Geometry check sheet. Reference: the model listing, model coordinates, mm. Face numbers are marked on the shaded views. A direction names the side the tool comes from. Coordinates: 2 decimals unless noted, no trailing zeros. Loops run counter-clockwise (first coordinate to the right, second up) from the corner with the lowest first, then second, coordinate; pieces in that order, holes last.
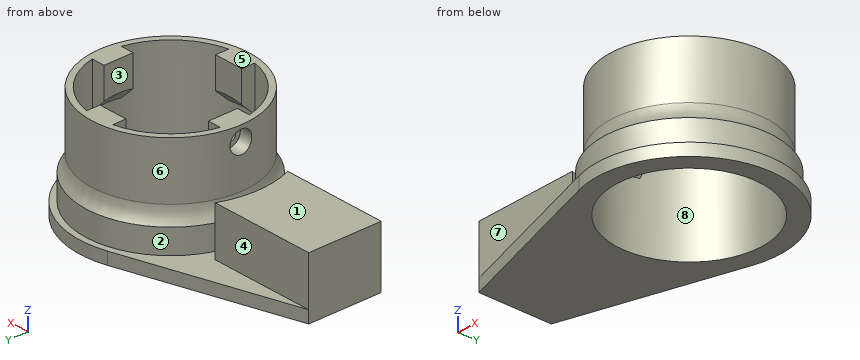
from build123d import *

# Parameters (mm, degrees)
ESQUISSE1_R                  = 30
BOSS_EXTRU_1_DEPTH           = 5
ESQUISSE6_R                  = 35
ESQUISSE6_R_2                = 30
BOSS_EXTRU_6_DEPTH           = 10
ESQUISSE7_R                  = 32.5
ESQUISSE7_R_2                = 30
BOSS_EXTRU_8_DEPTH           = 30
CONG_2_R                     = 10
BOSS_EXTRU_9_DEPTH           = 20
ESQUISSE9_W                  = 8
ESQUISSE9_H                  = 12
ESQUISSE9_W_2                = 12
ESQUISSE9_H_2                = 8
BOSS_EXTRU_10_DEPTH          = 12
CHANFREIN1_SIZE              = 6
ENL_V_MAT_EXTRU_1_REACH      = 86.89
ENL_V_MAT_EXTRU_1_END_RADIUS = 32.5
ESQUISSE10_R                 = 4.5
ESQUISSE12_R                 = 4.5
ESQUISSE12_R_2               = 2.6
BOSS_EXTRU_11_DEPTH          = 3


with BuildPart() as part:
    # Esquisse1 → Boss.-Extru.1 (new body)
    with BuildSketch(Plane.XY):
        with BuildLine():
            Line((-10.847469364, 35.896830061), (-80, 15))
            Line((-80, 15), (-80, -15))
            Line((-80, -15), (-10.847469364, -35.896830061))
            ThreePointArc((-10.847469364, -35.896830061), (37.5, 0), (-10.847469364, 35.896830061))
        make_face()
        Circle(ESQUISSE1_R, mode=Mode.SUBTRACT)
    extrude(amount=BOSS_EXTRU_1_DEPTH)

    # Esquisse6 → Boss.-Extru.6 (add)
    with BuildSketch(Plane.XY.offset(5)):
        Circle(ESQUISSE6_R)
        Circle(ESQUISSE6_R_2, mode=Mode.SUBTRACT)
    extrude(amount=BOSS_EXTRU_6_DEPTH)

    # Esquisse7 → Boss.-Extru.8 (add)
    with BuildSketch(Plane.XY.offset(15)):
        Circle(ESQUISSE7_R)
        Circle(ESQUISSE7_R_2, mode=Mode.SUBTRACT)
    extrude(amount=BOSS_EXTRU_8_DEPTH)

    # Congé2
    # the kernel refuses this fillet: 10 mm, written as the material it adds along each edge
    with BuildSketch(Plane(origin=(0, 0, 15), x_dir=(1, 0, 0), z_dir=(0, -1, 0))) as cong_2_piece_1:
        with BuildLine():
            CenterArc((42.5, 6.614378278), CONG_2_R, 180, 41.409622109)
            Line((32.5, 6.614378278), (32.3, 6.614378278))
            Line((32.3, 6.614378278), (32.3, 0))
            Line((32.3, 0), (32.5, -0.2))
            ThreePointArc((32.5, -0.2), (33.75, -0.2), (34.85, -0.132287566))
            Line((34.85, -0.132287566), (35, 0))
        make_face()
    revolve(axis=Axis((0, 0, 15), (0, 0, 1)))

    # Esquisse8 → Boss.-Extru.9 (add)
    with BuildSketch(Plane.XY.offset(5)):
        with BuildLine():
            Line((-80, 15), (-37.080992435, 15))
            ThreePointArc((-37.080992435, 15), (-40, 0), (-37.080992435, -15))
            Line((-37.080992435, -15), (-80, -15))
            Line((-80, -15), (-80, 15))
        make_face()
    extrude(amount=BOSS_EXTRU_9_DEPTH)

    # Esquisse9 → Boss.-Extru.10 (add)
    with BuildSketch(Plane.XY.offset(45)):
        with Locations((-27.941352507, 0)):
            Rectangle(ESQUISSE9_W, ESQUISSE9_H)
        with Locations((0, 27.941352507)):
            Rectangle(ESQUISSE9_W_2, ESQUISSE9_H_2)
        with Locations((27.941352507, 0)):
            Rectangle(ESQUISSE9_W, ESQUISSE9_H)
        with Locations((0, -27.941352507)):
            Rectangle(ESQUISSE9_W_2, ESQUISSE9_H_2)
    extrude(amount=-BOSS_EXTRU_10_DEPTH)

    # Chanfrein1
    # the kernel refuses this chamfer: 6 mm, written as the material it adds along each edge
    with BuildSketch(Plane(origin=(0, 0, 33), x_dir=(-0.6561519302770997, 0.75462881232672, 0), z_dir=(-0.75462881232672, -0.6561519302770997, 0))) as chanfrein1_piece_1_section:
        Polygon((30, CHANFREIN1_SIZE), (30 - CHANFREIN1_SIZE, 0), (30, 0), align=None)
    chanfrein1_piece_1 = revolve(axis=Axis((0, 0, 33), (0, 0, -1)), revolution_arc=82.01410645, mode=Mode.PRIVATE)
    chanfrein1_piece_1 = split(chanfrein1_piece_1, bisect_by=Plane(origin=(-6, 27.82841678, 31.008979001), z_dir=(1, 0, 0)), keep=Keep.TOP, mode=Mode.PRIVATE)
    chanfrein1_piece_1 = split(chanfrein1_piece_1, bisect_by=Plane(origin=(6, 27.82841678, 31.008979001), z_dir=(-1, 0, 0)), keep=Keep.TOP, mode=Mode.PRIVATE)
    chanfrein1_piece_1 = split(chanfrein1_piece_1, bisect_by=Plane(origin=(0, 23.941352507, 31.008979001), z_dir=(0, 1, 0)), keep=Keep.TOP, mode=Mode.PRIVATE)
    add(chanfrein1_piece_1)
    with BuildSketch(Plane(origin=(0, 0, 33), x_dir=(0.754635493716526, 0.6561442460490032, 0), z_dir=(-0.6561442460490032, 0.754635493716526, 0))) as chanfrein1_piece_2_section:
        Polygon((30, CHANFREIN1_SIZE), (30 - CHANFREIN1_SIZE, 0), (30, 0), align=None)
    chanfrein1_piece_2 = revolve(axis=Axis((0, 0, 33), (0, 0, -1)), revolution_arc=41.006469797, mode=Mode.PRIVATE)
    chanfrein1_piece_2 = split(chanfrein1_piece_2, bisect_by=Plane(origin=(27.828416771, 6, 31.008979004), z_dir=(0, -1, 0)), keep=Keep.TOP, mode=Mode.PRIVATE)
    chanfrein1_piece_2 = split(chanfrein1_piece_2, bisect_by=Plane(origin=(23.941352507, 3.002348554, 31.008979004), z_dir=(1, 0, 0)), keep=Keep.TOP, mode=Mode.PRIVATE)
    add(chanfrein1_piece_2)
    with BuildSketch(Plane(origin=(0, 0, 33), x_dir=(0.6561519302770998, -0.7546288123267199, 0), z_dir=(0.7546288123267199, 0.6561519302770998, 0))) as chanfrein1_piece_3_section:
        Polygon((30, CHANFREIN1_SIZE), (30 - CHANFREIN1_SIZE, 0), (30, 0), align=None)
    chanfrein1_piece_3 = revolve(axis=Axis((0, 0, 33), (0, 0, -1)), revolution_arc=82.01410645, mode=Mode.PRIVATE)
    chanfrein1_piece_3 = split(chanfrein1_piece_3, bisect_by=Plane(origin=(6, -27.82841678, 31.008979001), z_dir=(-1, 0, 0)), keep=Keep.TOP, mode=Mode.PRIVATE)
    chanfrein1_piece_3 = split(chanfrein1_piece_3, bisect_by=Plane(origin=(-6, -27.82841678, 31.008979001), z_dir=(1, 0, 0)), keep=Keep.TOP, mode=Mode.PRIVATE)
    chanfrein1_piece_3 = split(chanfrein1_piece_3, bisect_by=Plane(origin=(0, -23.941352507, 31.008979001), z_dir=(0, -1, 0)), keep=Keep.TOP, mode=Mode.PRIVATE)
    add(chanfrein1_piece_3)
    with BuildSketch(Plane(origin=(0, 0, 33), x_dir=(-0.7546288123267202, -0.6561519302770997, 0), z_dir=(0.6561519302770997, -0.7546288123267202, 0))) as chanfrein1_piece_4_section:
        Polygon((30, CHANFREIN1_SIZE), (30 - CHANFREIN1_SIZE, 0), (30, 0), align=None)
    chanfrein1_piece_4 = revolve(axis=Axis((0, 0, 33), (0, 0, -1)), revolution_arc=82.01410645, mode=Mode.PRIVATE)
    chanfrein1_piece_4 = split(chanfrein1_piece_4, bisect_by=Plane(origin=(-27.82841678, -6, 31.008979), z_dir=(0, 1, 0)), keep=Keep.TOP, mode=Mode.PRIVATE)
    chanfrein1_piece_4 = split(chanfrein1_piece_4, bisect_by=Plane(origin=(-27.82841678, 6, 31.008979), z_dir=(0, -1, 0)), keep=Keep.TOP, mode=Mode.PRIVATE)
    chanfrein1_piece_4 = split(chanfrein1_piece_4, bisect_by=Plane(origin=(-23.941352507, 0, 31.008979), z_dir=(-1, 0, 0)), keep=Keep.TOP, mode=Mode.PRIVATE)
    add(chanfrein1_piece_4)
    with BuildSketch(Plane(origin=(0, 0, 33), x_dir=(1, 0, 0), z_dir=(0, 1, 0))) as chanfrein1_piece_5_section:
        Polygon((30, CHANFREIN1_SIZE), (30 - CHANFREIN1_SIZE, 0), (30, 0), align=None)
    chanfrein1_piece_5 = revolve(axis=Axis((0, 0, 33), (0, 0, -1)), revolution_arc=41.006469797, mode=Mode.PRIVATE)
    chanfrein1_piece_5 = split(chanfrein1_piece_5, bisect_by=Plane(origin=(27.828416774, -6, 31.008979003), z_dir=(0, 1, 0)), keep=Keep.TOP, mode=Mode.PRIVATE)
    chanfrein1_piece_5 = split(chanfrein1_piece_5, bisect_by=Plane(origin=(23.941352507, -3.002348554, 31.008979003), z_dir=(1, 0, 0)), keep=Keep.TOP, mode=Mode.PRIVATE)
    add(chanfrein1_piece_5)

    # Enlèv. mat.-Extru.1: up to this cylinder (the profile starts inside it)
    enl_v_mat_extru_1_end = Plane(origin=(0, 0, 39), z_dir=(0, 0, -1)) * Cylinder(ENL_V_MAT_EXTRU_1_END_RADIUS, 239.78, mode=Mode.PRIVATE)
    # Esquisse10 → Enlèv. mat.-Extru.1 (cut, up to the surface)
    with BuildSketch(Plane(origin=(-23.941352507, 0, 0), x_dir=(0, 0, -1), z_dir=(1, 0, 0)), mode=Mode.PRIVATE) as enl_v_mat_extru_1_sk1:
        with Locations((-39, 0)):
            Circle(ESQUISSE10_R)
    enl_v_mat_extru_1_tool1 = extrude(enl_v_mat_extru_1_sk1.sketch, amount=-ENL_V_MAT_EXTRU_1_REACH, mode=Mode.PRIVATE) & enl_v_mat_extru_1_end
    add(enl_v_mat_extru_1_tool1.solids().sort_by_distance((-23.941353, 0, 39))[0], mode=Mode.SUBTRACT)

    # Esquisse12 → Boss.-Extru.11 (add)
    with BuildSketch(Plane(origin=(-23.941352507, 0, 0), x_dir=(0, 0, -1), z_dir=(1, 0, 0))):
        with Locations((-39, 0)):
            Circle(ESQUISSE12_R)
        with Locations((-39, 0)):
            Circle(ESQUISSE12_R_2, mode=Mode.SUBTRACT)
    extrude(amount=-BOSS_EXTRU_11_DEPTH)


solid = part.part
(1) Sectioned sample at B-B on z = 7. Record the cut outline in (x, y), and give its area (3 significant figures).
Findings:
outline: (-80, -15) - (-37.08, -15) arc R40 cw to (-37.08, 15) - (-80, 15) - close; circle Ø70 at (0, 0); hole circle Ø60 at (0, 0)
area: 2,250 mm2
(2) Access from +Z, -Z, +X, -X, +Y, -Y to the whole of each face (thin tool, end or side, straight path). Record for the marked faces 1, 2, 3 and 4.
Findings:
face 1: +Z, -X, +Y, -Y
face 2: +Z
face 3: +Z, -Z
face 4: +Z, -X, +Y
(3) Scan lines: L1, parallel to X at y = -10.5, z = 9; L2, parallel to Y at x = 0, z = 14; L3, parallel to X at y = -2, z = 23. Record each from-to range of solid material in increasing order.
Findings:
L1: x = -80 to -38.6, -33.39 to -28.1, 28.1 to 33.39
L2: y = -35 to -30, 30 to 35
L3: x = -80 to -39.95, -32.44 to -29.93, 29.93 to 32.44
(4) Sectioned sample at C-C on z = 39. Record the cut outline in (x, y), and give its area (3 significant figures).
Findings:
outline: (-32.19, -4.5) arc R32.5 ccw (long way) to (-32.19, 4.5) - (-26.94, 4.5) - (-26.94, 2.6) - (-23.94, 2.6) - (-23.94, 6) - (-29.39, 6) arc R30 cw to (-6, 29.39) - (-6, 23.94) - (6, 23.94) - (6, 29.39) arc R30 cw to (29.39, 6) - (23.94, 6) - (23.94, -6) - (29.39, -6) arc R30 cw to (6, -29.39) - (6, -23.94) - (-6, -23.94) - (-6, -29.39) arc R30 cw to (-29.39, -6) - (-23.94, -6) - (-23.94, -2.6) - (-26.94, -2.6) - (-26.94, -4.5) - close
area: 707 mm2
(5) Gauge pin test, flat ends, axial feed: pin 1 Ø6 at (x, z) = (-25.5, 40) entering from -Y; pin 2 Ø4.5 at (y, z) = (0, 41) entering from -X; pin 3 Ø2 at (x, y) = (-42, 18.5) entering from +Z. Record the tip position at first contact, or that the pin passes through.
Findings:
pin 1: stops at y = -23.45
pin 2: stops at x = -26.94
pin 3: stops at z = 5
(6) Sectioned sample at D-D on y = -25.5. State how many separate pieces and enclosed holes the cut face has, and give its area (3 significant figures).
Findings:
separate pieces: 3
enclosed holes: 0
area: 811 mm2
(7) Sectioned sample at A-A on x = 0. Record the cut outline in (y, z).
Findings:
outline: (-37.5, 0) - (-30, 0) - (-30, 27) - (-24, 33) - (-23.94, 33) - (-23.94, 45) - (-32.5, 45) - (-32.5, 21.61) arc R10 cw to (-35, 15) - (-35, 5) - (-37.5, 5) - close; (23.94, 33) - (24, 33) - (30, 27) - (30, 0) - (37.5, 0) - (37.5, 5) - (35, 5) - (35, 15) arc R10 cw to (32.5, 21.61) - (32.5, 45) - (23.94, 45) - close
(8) Draft check along Y on the marked faces 5, 6, 7 and 8. Enter one of: +Y half, -Y half, draft (parallel to the pull), parting line (faces both ways), or undercut.
Findings:
face 5: draft
face 6: parting line
face 7: -Y half
face 8: undercut
